Design review of the part built by this model. Coordinates are the model's own, in mm. Coordinates: 2 decimals unless noted, no trailing zeros. Loops run counter-clockwise (first coordinate to the right, second up) from the corner with the lowest first, then second, coordinate; pieces in that order, holes last. Notation, with made-up numbers: (4.25, 67) -> (11.25, 67) arc R26 cw to (11.25, 105) -> close; hole circle Ø5 at (86.25, 48). An arc over 180 degrees is marked (long way). One line per item, written item: value. Start each with the question number.
1. Add section C-C on z = 71. Write out the cut boundary in (x, y) (3 decimals), plus the area to 3 significant figures.
2. Insertion check: pin 1 (6 mm diameter, centred on y = -29.5, z = 134, fed in from +X); pin 2 (1.5 mm diameter, centred on y = -44, z = 109, fed in from -X); pin 3 (1 mm diameter, centred on y = 66.5, z = 78.5, fed in from +X). Each pin has a flat end and moves straight along its axis. Give the tip position at first contact, or say it passes through.
3. Add section D-D on z = 134. Write out the cut boundary in (x, y), plus the area to 3 significant figures.
4. Add section A-A on y = 0. Write out the cut boundary in (x, z).
5. For probe 1 along Y at (x, z) = (2, 110.5); probe 2 along Z at (x, y) = (89.5, 78.5), list the stretches that pass through material, from the lowest coordinate up.
```python
from build123d import *

# Parameters (mm, degrees)
SKETCH1_R           = 114.3
BOSS_EXTRUDE1_DEPTH = 114.3
SKETCH2_R           = 117.9068
SKETCH2_R_2         = 114.3
BOSS_EXTRUDE2_DEPTH = 30.48
SKETCH3_R           = 114.3
BOSS_EXTRUDE3_DEPTH = 5.08


with BuildPart() as part:
    # Sketch1 → Boss-Extrude1 (new body)
    with BuildSketch(Plane.XY):
        with BuildLine():
            ThreePointArc((-31.793446259, 122.3), (-48.357791931, 116.746037126), (-63.997797892, 108.960520786))
            Line((-63.997797892, 108.960520786), (-108.960520786, 63.997797892))
            ThreePointArc((-108.960520786, 63.997797892), (-116.746037126, 48.357791931), (-122.3, 31.793446259))
            Line((-122.3, 31.793446259), (-122.3, -31.793446259))
            ThreePointArc((-122.3, -31.793446259), (-116.746037126, -48.357791931), (-108.960520786, -63.997797892))
            Line((-108.960520786, -63.997797892), (-63.997797892, -108.960520786))
            ThreePointArc((-63.997797892, -108.960520786), (-48.357791931, -116.746037126), (-31.793446259, -122.3))
            Line((-31.793446259, -122.3), (31.793446259, -122.3))
            ThreePointArc((31.793446259, -122.3), (48.357791931, -116.746037126), (63.997797892, -108.960520786))
            Line((63.997797892, -108.960520786), (108.960520786, -63.997797892))
            ThreePointArc((108.960520786, -63.997797892), (116.746037126, -48.357791931), (122.3, -31.793446259))
            Line((122.3, -31.793446259), (122.3, 31.793446259))
            ThreePointArc((122.3, 31.793446259), (116.746037126, 48.357791931), (108.960520786, 63.997797892))
            Line((108.960520786, 63.997797892), (63.997797892, 108.960520786))
            ThreePointArc((63.997797892, 108.960520786), (48.357791931, 116.746037126), (31.793446259, 122.3))
            Line((31.793446259, 122.3), (-31.793446259, 122.3))
        make_face()
        Circle(SKETCH1_R, mode=Mode.SUBTRACT)
    extrude(amount=BOSS_EXTRUDE1_DEPTH)

    # Sketch2 → Boss-Extrude2 (add)
    with BuildSketch(Plane.XY.offset(114.3)):
        with Locations(Location((0, 0, 0), (0, 0, 180))):
            Circle(SKETCH2_R)
        Circle(SKETCH2_R_2, mode=Mode.SUBTRACT)
    extrude(amount=BOSS_EXTRUDE2_DEPTH)

    # Sketch3 → Boss-Extrude3 (add)
    with BuildSketch(Plane.XY.offset(144.78)):
        with BuildLine():
            Line((122.3, -31.793446259), (122.3, 31.793446259))
            ThreePointArc((122.3, 31.793446259), (116.746037126, 48.357791931), (108.960520786, 63.997797892))
            Line((108.960520786, 63.997797892), (63.997797892, 108.960520786))
            ThreePointArc((63.997797892, 108.960520786), (48.357791931, 116.746037126), (31.793446259, 122.3))
            Line((31.793446259, 122.3), (-31.793446259, 122.3))
            ThreePointArc((-31.793446259, 122.3), (-48.357791931, 116.746037126), (-63.997797892, 108.960520786))
            Line((-63.997797892, 108.960520786), (-108.960520786, 63.997797892))
            ThreePointArc((-108.960520786, 63.997797892), (-116.746037126, 48.357791931), (-122.3, 31.793446259))
            Line((-122.3, 31.793446259), (-122.3, -31.793446259))
            ThreePointArc((-122.3, -31.793446259), (-116.746037126, -48.357791931), (-108.960520786, -63.997797892))
            Line((-108.960520786, -63.997797892), (-63.997797892, -108.960520786))
            ThreePointArc((-63.997797892, -108.960520786), (-48.357791931, -116.746037126), (-31.793446259, -122.3))
            Line((-31.793446259, -122.3), (31.793446259, -122.3))
            ThreePointArc((31.793446259, -122.3), (48.357791931, -116.746037126), (63.997797892, -108.960520786))
            Line((63.997797892, -108.960520786), (108.960520786, -63.997797892))
            ThreePointArc((108.960520786, -63.997797892), (116.746037126, -48.357791931), (122.3, -31.793446259))
        make_face()
        Circle(SKETCH3_R, mode=Mode.SUBTRACT)
    extrude(amount=BOSS_EXTRUDE3_DEPTH)


solid = part.part
```
Worked answers:
1. outline: (-122.3, -31.793) arc R126.365 ccw to (-108.961, -63.998) -> (-63.998, -108.961) arc R126.365 ccw to (-31.793, -122.3) -> (31.793, -122.3) arc R126.365 ccw to (63.998, -108.961) -> (108.961, -63.998) arc R126.365 ccw to (122.3, -31.793) -> (122.3, 31.793) arc R126.365 ccw to (108.961, 63.998) -> (63.998, 108.961) arc R126.365 ccw to (31.793, 122.3) -> (-31.793, 122.3) arc R126.365 ccw to (-63.998, 108.961) -> (-108.961, 63.998) arc R126.365 ccw to (-122.3, 31.793) -> close; hole circle Ø228.6 at (0, 0)
1. area: 7,740 mm²
2. pin 1: stops at x = 114.89
2. pin 2: stops at x = -118.73
2. pin 3: stops at x = 106.96
3. outline: circle Ø235.81 at (0, 0); hole circle Ø228.6 at (0, 0)
3. area: 2,630 mm²
4. outline: (-122.3, 0) -> (-114.3, 0) -> (-114.3, 149.86) -> (-122.3, 149.86) -> (-122.3, 144.78) -> (-117.91, 144.78) -> (-117.91, 114.3) -> (-122.3, 114.3) -> close; (114.3, 0) -> (122.3, 0) -> (122.3, 114.3) -> (117.91, 114.3) -> (117.91, 144.78) -> (122.3, 144.78) -> (122.3, 149.86) -> (114.3, 149.86) -> close
5. probe 1: y = -122.3 to -114.28, 114.28 to 122.3
5. probe 2: z = 0 to 114.3, 144.78 to 149.86
